Design review of the part built by this model. Coordinates are the model's own, in mm. A direction names the side the tool comes from. Coordinates: 2 decimals unless noted, no trailing zeros. Loops run counter-clockwise (first coordinate to the right, second up) from the corner with the lowest first, then second, coordinate; pieces in that order, holes last. Notation, with made-up numbers: M 0,16 L 42,16 A22 ccw 42,38 Z; hole C -0.5,-35.75 d10. An arc over 180 degrees is marked long. Write item = value, one per line. Start each with the question number.
from build123d import *
from OCP.BRepFilletAPI import BRepFilletAPI_MakeChamfer

# Parameters (mm, degrees)
FILLET1_R                          = 3.175
M4_CIRPATTERN1_COUNT               = 2
SKETCH6_R                          = 15.0749
F_0_88_FEEDTHRU_CUT_EXTRUDE2_DEPTH = 12.7
SKETCH7_R                          = 12.827
F_0_88_FEEDTHRU_CUT_EXTRUDE3_DEPTH = 88.078738909
SKETCH8_R                          = 19.05
F_1_5_FEEDTHRU_CUT_EXTRUDE4_DEPTH  = 12.7
SKETCH9_R                          = 17.526
F_1_5_FEEDTHRU_CUT_EXTRUDE5_DEPTH  = 88.078738909
M27X3_TAPPED_HOLE1_D               = 25
M27X3_TAPPED_HOLE1_DEPTH           = 12.7
M4X0_7_TAPPED_HOLE1_D              = 3.3
M4X0_7_TAPPED_HOLE1_DEPTH          = 12.10056
M4X0_7_TAPPED_HOLE1_TIP            = 0.991420021
CHAMFER1_SIZE                      = 0.79375
FILLET2_R                          = 0.254
CHAMFER2_SIZE                      = 1.27
CHAMFER2_SIZE2                     = 0.340295474


with BuildPart() as part:
    # Sketch1 → Revolve1 (revolve)
    with BuildSketch(Plane.XY, mode=Mode.PRIVATE) as revolve1_sk:
        Polygon((52.7431, 21.954), (52.7431, 29.8788), (17, 29.8788), (0, 29.8788), (0, 52.1038), (60.325, 52.1038), (60.325, 42.5788), (57.1246, 42.5788), (57.1246, 29.8788), (54.3306, 29.8788), (54.3306, 25.129), (57.1246, 25.129), (57.1246, 21.954), align=None)
    revolve(revolve1_sk.sketch.rotate(Axis((0, 0, 0), (0, 1, 0)), 90), axis=Axis((0, 0, 0), (0, 1, 0)))

    # Fillet1
    fillet1_edges = [part.edges().sort_by_distance(p)[0] for p in [
        (0, 29.8788, 52.7431),
    ]]
    fillet(fillet1_edges, radius=FILLET1_R)

    # Sketch5 → Tapped Hole for M4x0.7 Helicoil1 (revolve, cut)
    with BuildSketch(Plane(origin=(57.1246, 34.9588, 0), x_dir=(0, 0, -1), z_dir=(0, 1, 0))):
        Polygon((0, 0), (0, 11.4624473), (2.1, 10.20064), (2.1, 0), align=None)
    tapped_hole_for_m4x0_7_helicoil1 = revolve(axis=Axis((63.4746, 34.9588, 0), (-1, 0, 0)), mode=Mode.SUBTRACT)

    # M4 CirPattern1: Tapped Hole for M4x0.7 Helicoil1 ×2 about axis
    m4_cirpattern1_axis = Axis((0, 0, 0), (0, -1, 0))
    for i in range(1, M4_CIRPATTERN1_COUNT):
        add(tapped_hole_for_m4x0_7_helicoil1.rotate(m4_cirpattern1_axis, i * 360 / M4_CIRPATTERN1_COUNT), mode=Mode.SUBTRACT)

    # Sketch6 → 0.88 feedthru Cut-Extrude2 (cut)
    with BuildSketch(Plane(origin=(0, 52.1038, 0), x_dir=(1, 0, 0), z_dir=(0, 1, 0))):
        with Locations(Location((0, 38.89375, 0), (0, 0, 270))):
            Circle(SKETCH6_R)
        with Locations(Location((34.652531078, 17.661423469, 0), (0, 0, 270))):
            Circle(SKETCH6_R)
        with Locations(Location((-34.652531078, 17.661423469, 0), (0, 0, 270))):
            Circle(SKETCH6_R)
        with Locations(Location((31.471021727, -22.85385264, 0), (0, 0, 270))):
            Circle(SKETCH6_R)
    extrude(amount=-F_0_88_FEEDTHRU_CUT_EXTRUDE2_DEPTH, mode=Mode.SUBTRACT)

    # Sketch7 → 0.88 feedthru Cut-Extrude3 (cut, through all)
    with BuildSketch(Plane(origin=(0, 39.4038, 0), x_dir=(1, 0, 0), z_dir=(0, 1, 0))):
        with Locations(Location((0, 38.89375, 0), (0, 0, 270))):
            Circle(SKETCH7_R)
        with Locations(Location((34.652531078, 17.661423469, 0), (0, 0, 270))):
            Circle(SKETCH7_R)
        with Locations(Location((-34.652531078, 17.661423469, 0), (0, 0, 270))):
            Circle(SKETCH7_R)
        with Locations(Location((31.471021727, -22.85385264, 0), (0, 0, 270))):
            Circle(SKETCH7_R)
    extrude(amount=-F_0_88_FEEDTHRU_CUT_EXTRUDE3_DEPTH, mode=Mode.SUBTRACT)

    # Sketch8 → 1.5 feedthru Cut-Extrude4 (cut)
    with BuildSketch(Plane(origin=(0, 52.1038, 0), x_dir=(1, 0, 0), z_dir=(0, 1, 0))):
        with Locations(Location((-18.246530612, -29.779518895, 0), (0, 0, 270))):
            Circle(SKETCH8_R)
    extrude(amount=-F_1_5_FEEDTHRU_CUT_EXTRUDE4_DEPTH, mode=Mode.SUBTRACT)

    # Sketch9 → 1.5 feedthru Cut-Extrude5 (cut, through all)
    with BuildSketch(Plane(origin=(0, 39.4038, 0), x_dir=(1, 0, 0), z_dir=(0, 1, 0))):
        with Locations(Location((-18.246530612, -29.779518895, 0), (0, 0, 270))):
            Circle(SKETCH9_R)
    extrude(amount=-F_1_5_FEEDTHRU_CUT_EXTRUDE5_DEPTH, mode=Mode.SUBTRACT)

    # M27x3 Tapped Hole1
    with Locations(Plane(origin=(0, 29.8788, 0), x_dir=(-1, 0, 0), z_dir=(0, -1, 0))):
        with Locations((0, 0)):
            Hole(M27X3_TAPPED_HOLE1_D / 2, depth=M27X3_TAPPED_HOLE1_DEPTH)

    # M4x0.7 Tapped Hole1
    with Locations(Plane(origin=(0, 29.8788, 0), x_dir=(-1, 0, 0), z_dir=(0, -1, 0))):
        with Locations((-22.393469388, 36.547591371), (42.39132394, -6.337946111), (-13.602834619, -40.646731684)):
            Hole(M4X0_7_TAPPED_HOLE1_D / 2, depth=M4X0_7_TAPPED_HOLE1_DEPTH)
            with Locations((0, 0, -(M4X0_7_TAPPED_HOLE1_DEPTH + M4X0_7_TAPPED_HOLE1_TIP / 2))):  # 118° drill point
                Cone(0, M4X0_7_TAPPED_HOLE1_D / 2, M4X0_7_TAPPED_HOLE1_TIP, mode=Mode.SUBTRACT)

    # Chamfer1
    chamfer1_edges = [part.edges().sort_by_distance(p)[0] for p in [
        (0, 21.954, 57.1246),
    ]]
    chamfer(chamfer1_edges, length=CHAMFER1_SIZE)

    # Fillet2
    fillet2_edges = [part.edges().sort_by_distance(p)[0] for p in [
        (0, 29.8788, 54.3306),
        (0, 25.129, 54.3306),
    ]]
    fillet(fillet2_edges, radius=FILLET2_R)

    # Chamfer2: one chamfer whose edges measure the first distance from different faces: ONE call of the kernel's chamfer builder (chamfer() names one face for all edges)
    chamfer2_edges_1 = [part.edges().sort_by_distance(p)[0] for p in [
        (0, 52.1038, -53.96865),
    ]]
    chamfer2_side_1 = [part.faces().sort_by_distance(p)[0] for p in [
        (0, 45.7538, -53.96865),
    ]]
    chamfer2_edges_2 = [part.edges().sort_by_distance(p)[0] for p in [
        (31.471021727, 52.1038, 7.77895264),
    ]]
    chamfer2_side_2 = [part.faces().sort_by_distance(p)[0] for p in [
        (31.471021727, 45.7538, 7.77895264),
    ]]
    chamfer2_edges_3 = [part.edges().sort_by_distance(p)[0] for p in [
        (-34.652531078, 52.1038, -32.736323469),
    ]]
    chamfer2_side_3 = [part.faces().sort_by_distance(p)[0] for p in [
        (-34.652531078, 45.7538, -32.736323469),
    ]]
    chamfer2_edges_4 = [part.edges().sort_by_distance(p)[0] for p in [
        (34.652531078, 52.1038, -32.736323469),
    ]]
    chamfer2_side_4 = [part.faces().sort_by_distance(p)[0] for p in [
        (34.652531078, 45.7538, -32.736323469),
    ]]
    chamfer2_edges_5 = [part.edges().sort_by_distance(p)[0] for p in [
        (-18.246530612, 52.1038, 10.729518895),
    ]]
    chamfer2_side_5 = [part.faces().sort_by_distance(p)[0] for p in [
        (-18.246530612, 45.7538, 10.729518895),
    ]]
    chamfer2 = BRepFilletAPI_MakeChamfer(part.part.solid().wrapped)
    for e in chamfer2_edges_1:
        chamfer2.Add(CHAMFER2_SIZE, CHAMFER2_SIZE2, e.wrapped, chamfer2_side_1[0].wrapped)  # the first distance lies on this face
    for e in chamfer2_edges_2:
        chamfer2.Add(CHAMFER2_SIZE, CHAMFER2_SIZE2, e.wrapped, chamfer2_side_2[0].wrapped)  # the first distance lies on this face
    for e in chamfer2_edges_3:
        chamfer2.Add(CHAMFER2_SIZE, CHAMFER2_SIZE2, e.wrapped, chamfer2_side_3[0].wrapped)  # the first distance lies on this face
    for e in chamfer2_edges_4:
        chamfer2.Add(CHAMFER2_SIZE, CHAMFER2_SIZE2, e.wrapped, chamfer2_side_4[0].wrapped)  # the first distance lies on this face
    for e in chamfer2_edges_5:
        chamfer2.Add(CHAMFER2_SIZE, CHAMFER2_SIZE2, e.wrapped, chamfer2_side_5[0].wrapped)  # the first distance lies on this face
    add(Compound.cast(chamfer2.Shape()), mode=Mode.REPLACE)


solid = part.part
Q1. To check wall thickness, follow line 1 (Y direction, x = 54, z = -16); line 2 (Z direction, x = 9.5, y = 41.5); line 3 (Z direction, x = 10, y = 32). State the ranges of each line that lie inside material, in increasing order. Write a range as from..to.
Q2. Add section A-A on y = 44.5. State the section outline as (x, z) points (3 decimals).
Q3. For faces 1 (the face through (0.663, 45.199, -53.954)), 2 (the face through (47.37, 34.29, -19.33)), 3 (the face through (-15.84, 24.36, -50.31)), list the 3-axis set-ups (+Z, -Z, +X, -X, +Y, -Y) from which the entire face can be reached by the end or side of a thin tool; tool diameter is ignored.
Q4. Clearance check with flat-ended pins moving along their axes: P1, Ø5.5, axis at x = 22.39, z = -36.55, coming from the -Y side; P2, Ø4, axis at y = 34.96, z = 0, coming from the +X side; P3, Ø23, axis at x = 31.47, z = 22.85, coming from the -Y side; P4, Ø5, axis at y = 25.5, z = -1.5, coming from the -X side. State where each tip first meets the part, or that it passes through.
Q5. Mouldability with a two-part tool opening along X and no side actions: class faces 4 (the face through (-29.838, 45.199, 14.662)), 5 (the face through (16.4, 21.954, 50.3)), 6 (the face through (45.9, 34.7, 0.3)) as released by +X, released by -X, zero draft, split by the parting line, or undercut.
Q6. Add section B-B on x = 29. Give the number of separate pieces and of enclosed holes in the cut face, plus the area to 3 significant figures.
Values follow:
q1.line_1 = 21.95..25.13, 29.88..52.1
q1.line_2 = -56.33..-50.6, -27.19..-8.12, 8.12..56.33
q1.line_3 = -56.24..-46.93, -30.86..-7.5, 7.5..56.24
q2.outline = C 0,0 d120.65; hole C -34.653,-17.661 d30.15; hole C -18.247,29.78 d38.1; hole C 0,-38.894 d30.15; hole C 31.471,22.854 d30.15; hole C 34.653,-17.661 d30.15
q3.face_1 = +Y
q3.face_2 = +Y, -Y
q3.face_3 = -Y
q4.P1 = 29.88
q4.P2 = 46.86
q4.P3 = through
q4.P4 = -57.12
q5.face_4 = undercut
q5.face_5 = zero draft
q5.face_6 = released by +X
q6.separate_pieces = 3
q6.enclosed_holes = 0
q6.area = 1,120 mm2
